Job drawing, mm, ordinate dimensions from the low corner. One solid piece. Coordinates: 2 decimals unless noted, no trailing zeros. Write each loop counter-clockwise with the first axis right and the second up, starting at its lowest first coordinate (ties: lowest second). Pieces come first, ordered by that corner, then holes. Notation, with made-up numbers: (12.25, 10) -> (35.25, 10) arc R20 cw to (35.25, 29) -> close; hole circle Ø2 at (88.25, 37.25). An arc over 180 degrees is marked (long way). Answer as a JSON object with one key per item and string values. Group by question number.
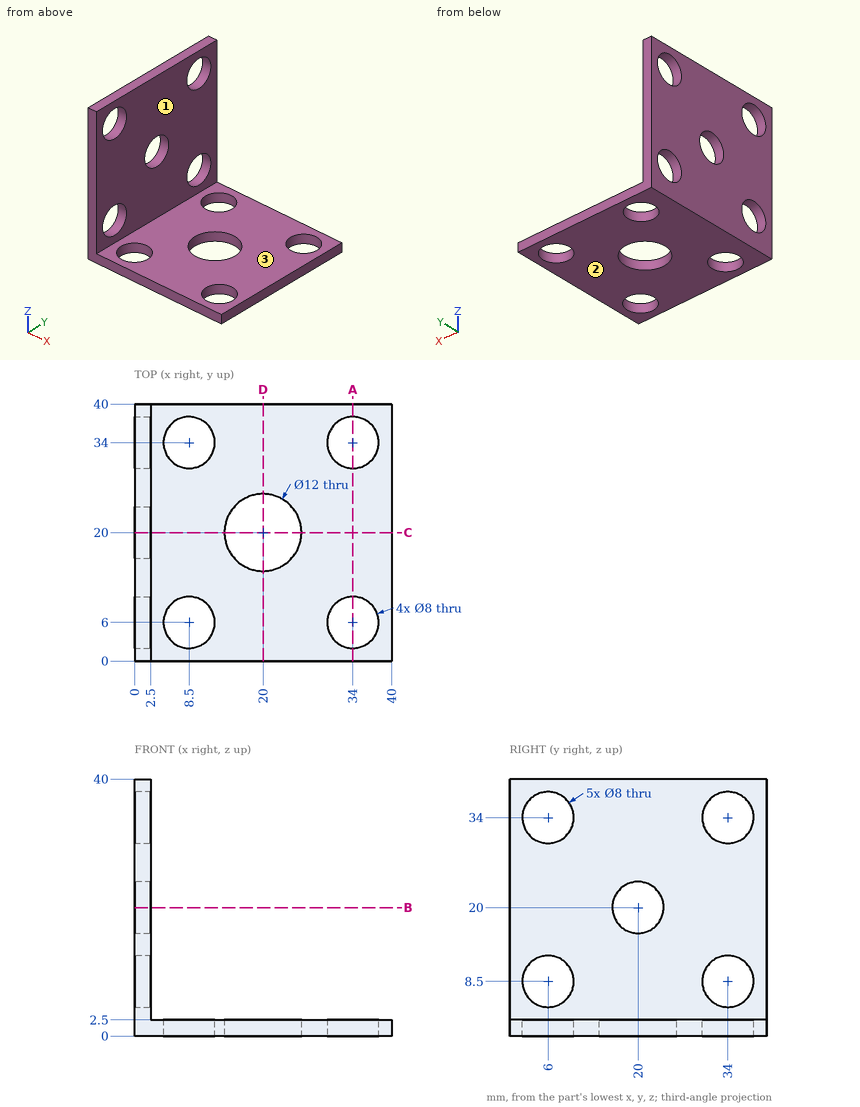
(1) Pull direction Z, two halves, no side cores. Call the marked faces 1, 2 and 3: released by +Z, released by -Z, zero draft, split by the parting line, or undercut.
(2) Cut at D-D on x = 20. List the corners of the cut face in (y, z), plus the area to 3 significant figures.
(3) Cut at C-C on y = 20. List the corners of the cut face in (x, z).
(4) Cut at A-A on x = 34. List the corners of the cut face in (y, z).
(5) Pin check, flat tips, straight feed: pin 1 (9 mm diameter, centred on x = 8.5, y = 34, fed in from +Z); pin 2 (4 mm diameter, centred on y = 9, z = 16, fed in from +X); pin 3 (10.5 mm diameter, centred on y = 6, z = 8.5, fed in from -X). Stop position of each tip, or through.
(6) Wall check: probe 1 along Y at (x, z) = (8.5, 1.55); probe 2 along Z at (x, y) = (1.85, 34). Give the ranges that are in metal, low to high.
(7) Cut at B-B on z = 20. List the corners of the cut face in (x, y), plus the area to 3 significant figures.
Results found:
{
 "1": {"face 1": "zero draft", "face 2": "released by -Z", "face 3": "released by +Z"},
 "2": {"outline": "(0, 0) -> (14, 0) -> (14, 2.5) -> (0, 2.5) -> close; (26, 0) -> (40, 0) -> (40, 2.5) -> (26, 2.5) -> close", "area": "70.0 mm²"},
 "3": {"outline": "(0, 0) -> (14, 0) -> (14, 2.5) -> (2.5, 2.5) -> (2.5, 16) -> (0, 16) -> close; (0, 24) -> (2.5, 24) -> (2.5, 40) -> (0, 40) -> close; (26, 0) -> (40, 0) -> (40, 2.5) -> (26, 2.5) -> close"},
 "4": {"outline": "(0, 0) -> (2, 0) -> (2, 2.5) -> (0, 2.5) -> close; (10, 0) -> (30, 0) -> (30, 2.5) -> (10, 2.5) -> close; (38, 0) -> (40, 0) -> (40, 2.5) -> (38, 2.5) -> close"},
 "5": {"pin 1": "stops at z = 2.5", "pin 2": "stops at x = 2.5", "pin 3": "stops at x = 0"},
 "6": {"probe 1": "y = 0 to 2, 10 to 30, 38 to 40", "probe 2": "z = 0 to 4.5, 12.5 to 30, 38 to 40"},
 "7": {"outline": "(0, 0) -> (2.5, 0) -> (2.5, 16) -> (0, 16) -> close; (0, 24) -> (2.5, 24) -> (2.5, 40) -> (0, 40) -> close", "area": "80.0 mm²"}
}
